Autodesk Fusion 360 part; units mm, degrees
sketch "Sketch1" plane through (0, 0, 0) normal (0, 1, 0) x (1, 0, 0)
  line L0 (4.5, 1.6) -> (-4.5, 1.6)
  line L1 (-4.5, 0.1) -> (-4.5, -0.1)
  line L2 (-3, -1.6) -> (3, -1.6)
  line L3 (4.5, -0.1) -> (4.5, 0.1)
  line L4 (4.5, 1.6) -> (-4.5, -1.6) construction
  line L5 (-4.5, 1.6) -> (4.5, -1.6) construction
  arc A0 (-4.5, -0.1) -> (-3, -1.6) centre (-3, -0.1) ccw
  arc A1 (3, -1.6) -> (4.5, -0.1) centre (3, -0.1) ccw
  line L6 (3, 1.6) -> (-3, 1.6)
  arc A2 (-3, 1.6) -> (-4.5, 0.1) centre (-3, 0.1) ccw
  arc A3 (4.5, 0.1) -> (3, 1.6) centre (3, 0.1) ccw
  line L7 (4.5, 1.6) -> (4.5, 0)
  line L8 (-4.5, 1.6) -> (-4.5, 0)
  line L9 (-5.25, 3.2) -> (5.25, 3.2)
  line L10 (5.25, 3.2) -> (5.25, 1.6)
  line L11 (5.25, 1.6) -> (-5.25, 1.6)
  line L12 (-5.25, 1.6) -> (-5.25, 3.2)
  point P0 (0, 1.6)
  point P1 (0, 1.6)
  dimension "d5" = 9
  dimension "d6" = 3.2
  dimension "d8" = 1.5
  dimension "d11" = 1.5
  dimension "d12" = 10.5
  dimension "d13" = 1.6
extrude "Extrude1" add sketch "Sketch1" along normal blind 10 contours L0 L1 L2 L3 A0 A1 L6 A2 A3 L7 L8 L11
extrude "Extrude2" add sketch "Sketch1" along normal blind 8.5 from surface at 1.5 contours L0 A3 L7 L11 | L0 L6 L9 L10 L11 L12 | L0 A2 L8 L11
move_face "OffsetFaces1" offset 0.3 12 faces at (4.4983, 6.6667, 0.1714) (-1, 3.3333, 1.6) (-3.0714, 6.6667, 1.5983) (-4.5, 7.1667, -0.5333) (-4.75, 4.3333, -1.6) (-5.25, 4.3333, -2.1333) (4.5, 7.1667, -0.5333) (3.0714, 1, -1.5983) (1, 0.5, -1.6) (-4.3926, 1, -0.6575) (5, 4.3333, -1.6) (5.25, 4.3333, -2.6667)
equation "usb_c_width = 9 mm"
equation "usb_c_height = 3.2 mm"
equation "pcb_thickness = 1.6 mm"
equation "pcb_width = 10.5 mm"
equation "d5 = usb_c_width"
equation "d6 = usb_c_height"
equation "usb_c_fillet = 1.5 mm"
equation "d8 = usb_c_fillet"
equation "d11 = usb_c_fillet"
equation "d12 = pcb_width"
equation "d13 = pcb_thickness"
Can you work these out from the model? Positions are in its coordinate system, mm. A direction names the side the tool comes from. Coordinates: 2 decimals unless noted, no trailing zeros. Loops run counter-clockwise (first coordinate to the right, second up) from the corner with the lowest first, then second, coordinate; pieces in that order, holes last. Notation, with made-up numbers: (54, 40.5) - (77, 40.5) arc R24 cw to (77, 72.5) - close; hole circle Ø1 at (70.25, -4). An arc over 180 degrees is marked (long way). Put each result on its own line as item: value. Start each with the question number.
Item 1: Suppose I cut it at B-B (y = 2.5). Please give me the cut outline in (x, z).
Item 2: If I drill on line 1 along Y through (x, z) = (-2.5, -2.5); line 2 along Z through (x, y) = (2.75, 0.5); line 3 along X through (y, z) = (3.75, 1.65), over which ranges is the centre line in solid material (lowest first)?
Item 3: Suppose I cut it at A-A (x = 0.5). Please give me the cut outline in (y, z).
Item 4: For pin 1 (1.5 mm diameter, centred on y = 5, z = -0.5, fed in from +X), with a flat end and sliding along its axis, tell me the tip position at first contact or that it passes through.
Item 5: Suppose I cut it at D-D (z = -1.7). Please give me the cut outline in (x, y), and give its area (3 significant figures).
Item 6: Which directions (+Z, -Z, +X, -X, +Y, -Y) give clear straight access to the entire face, cutting with the end or side of a thin tool? Please do faces 1 (the face through (-4.287, 0.74, -1.359)), 2 (the face through (4.8, 5, -1)), 3 (the face through (0, 1, -1.9)), 4 (the face through (4.259, 0.74, -1.387)), 5 (the face through (-4.8, 5, -1)).
Here are the results:
1. outline: (-5.55, -3.2) - (5.55, -3.2) - (5.55, -1.3) - (4.8, -1.3) - (4.8, 0.1) arc R1.8 ccw to (3, 1.9) - (-3, 1.9) arc R1.8 ccw to (-4.8, 0.1) - (-4.8, -1.3) - (-5.55, -1.3) - close
2. line 1: 1.5 to 10
2. line 2: -1.9 to 1.9
2. line 3: -3.92 to 3.92
3. outline: (0, -1.9) - (1.5, -1.9) - (1.5, -3.2) - (10, -3.2) - (10, 1.9) - (0, 1.9) - close
4. pin 1: x = 4.8
5. outline: (-5.55, 1.5) - (-3.82, 1.5) - (-3.82, 0) - (3.82, 0) - (3.82, 1.5) - (5.55, 1.5) - (5.55, 10) - (-5.55, 10) - close
5. area: 106 mm²
6. face 1: -Z, -X, -Y
6. face 2: +Z, +X, +Y, -Y
6. face 3: -Z, +X, -X, -Y
6. face 4: -Z, +X, -Y
6. face 5: +Z, -X, +Y, -Y
